Verification items for the finished model (mm, model axes). A direction names the side the tool comes from. Round coordinates to 2 decimals unless told otherwise and drop trailing zeros. Loops run counter-clockwise (first coordinate to the right, second up) from the corner with the lowest first, then second, coordinate; pieces in that order, holes last. Notation, with made-up numbers: M -12,12 L 38,12 A18 cw 38,28 Z; hole C -25,-19.75 d1. An arc over 180 degrees is marked long. Write item = value, one per line. Start each with the question number.
from build123d import *

# Parameters (mm, degrees)
BOSS_EXTRUDE1_DEPTH      = 46
SKETCH4_R                = 2.5
CUT_EXTRUDE2_DEPTH       = 49.124837662
CUT_EXTRUDE1_DEPTH       = 49.124837662
FILLET1_R                = 2
CIRPATTERN1_COUNT        = 4
FILLET1_OF_CIRPATTERN1_R = 2


with BuildPart() as part:
    # Sketch1 → Boss-Extrude1 (new body)
    with BuildSketch(Plane(origin=(0, 0, 0), x_dir=(1, 0, 0), z_dir=(0, 1, 0))):
        with BuildLine():
            Line((8.5, 10), (-8.5, 10))
            ThreePointArc((-8.5, 10), (-9.560660172, 9.560660172), (-10, 8.5))
            Line((-10, 8.5), (-10, -8.5))
            ThreePointArc((-10, -8.5), (-9.560660172, -9.560660172), (-8.5, -10))
            Line((-8.5, -10), (8.5, -10))
            ThreePointArc((8.5, -10), (9.560660172, -9.560660172), (10, -8.5))
            Line((10, -8.5), (10, 8.5))
            ThreePointArc((10, 8.5), (9.560660172, 9.560660172), (8.5, 10))
        make_face()
    extrude(amount=BOSS_EXTRUDE1_DEPTH)

    # Sketch4 → Cut-Extrude2 (cut, through all)
    with BuildSketch(Plane(origin=(0, 0, 0), x_dir=(1, 0, 0), z_dir=(0, 1, 0))):
        with Locations(Location((0, 0, 0), (0, 0, 270))):
            Circle(SKETCH4_R)
    extrude(amount=CUT_EXTRUDE2_DEPTH, mode=Mode.SUBTRACT)

    # Sketch2 → Cut-Extrude1 (cut, through all)
    with BuildSketch(Plane.XZ):
        Polygon((-3.6, -10), (-3.6, -9.5), (-3.1, -9.5), (-3.1, -8.2), (-5.5, -8.2), (-5.5, -6.560660172), (-2.839339828, -3.9), (2.839339828, -3.9), (5.5, -6.560660172), (5.5, -8.2), (3.1, -8.2), (3.1, -9.5), (3.6, -9.5), (3.6, -10), align=None)
    cut_extrude1 = extrude(amount=-CUT_EXTRUDE1_DEPTH, mode=Mode.SUBTRACT)

    # Fillet1
    fillet1_edges = [part.edges().sort_by_distance(p)[0] for p in [
        (-2.839339828, 23, -3.9),
        (2.839339828, 23, -3.9),
    ]]
    fillet(fillet1_edges, radius=FILLET1_R)

    # CirPattern1: Cut-Extrude1 ×4 about axis
    cirpattern1_axis = Axis((0, 0, 0), (0, 1, 0))
    for i in range(1, CIRPATTERN1_COUNT):
        add(cut_extrude1.rotate(cirpattern1_axis, i * 360 / CIRPATTERN1_COUNT), mode=Mode.SUBTRACT)

    # Fillet1 of CirPattern1
    fillet1_of_cirpattern1_edges = [part.edges().sort_by_distance(p)[0] for p in [
        (-3.9, 23, 2.839339828),
        (-3.9, 23, -2.839339828),
        (2.839339828, 23, 3.9),
        (-2.839339828, 23, 3.9),
        (3.9, 23, -2.839339828),
        (3.9, 23, 2.839339828),
    ]]
    fillet(fillet1_of_cirpattern1_edges, radius=FILLET1_OF_CIRPATTERN1_R)


solid = part.part
1. Tool access check on faces 4 (the cylindrical face through (4.05, 23.32, 2.77)), 5 (the flat face through (3.1, 23, 9)), 6 (the flat face through (-3.9, 23, 0)), 7 (the flat face through (9, 23, 3.1)). Record the directions out of +Z, -Z, +X, -X, +Y, -Y that give a thin tool (end or side, any length) a straight path to the whole face; none if there is none.
2. Thickness scan on line 1 (Z direction, x = 0, y = 28.5); line 2 (X direction, y = 24, z = -7.25). Record the ranges inside material, lowest first.
3. Section check B-B, the plane x = 0. Enter the section's corners in (y, z), and give its area (3 significant figures).
4. Section check A-A, the plane z = 0. Enter the section's corners in (x, y), and give its area (3 significant figures).
5. Mould release check, pull along Z, two halves, no side actions. Record for faces 1 (the flat face through (-10, 23, 6)), 2 (the cylindrical face through (2.77, 23.32, -4.05)), 3 (the flat face through (0, 23, -3.9)): pulls with the +Z half, pulls with the -Z half, needs draft (parallel to the pull), parting line crosses it, or undercut.
6. Gauge pin test, flat ends, axial feed: P1, Ø1.2, axis at x = 0, y = 12.5, coming from the -Z side; P2, Ø2, axis at y = 25, z = 0.5, coming from the +X side; P3, Ø0.6, axis at x = 3, y = 18.5, coming from the -Z side. Record the tip position at first contact, or that the pin passes through.
Computed values:
q1.face_4 = +Y, -Y
q1.face_5 = +Z, +Y, -Y
q1.face_6 = -X, +Y, -Y
q1.face_7 = +X, +Y, -Y
q2.line_1 = -3.9 to -2.5, 2.5 to 3.9
q2.line_2 = -10 to -5.5, 5.5 to 10
q3.outline = M 0,-3.9 L 46,-3.9 L 46,-2.5 L 0,-2.5 Z; M 0,2.5 L 46,2.5 L 46,3.9 L 0,3.9 Z
q3.area = 129 mm2
q4.outline = M -3.9,0 L -2.5,0 L -2.5,46 L -3.9,46 Z; M 2.5,0 L 3.9,0 L 3.9,46 L 2.5,46 Z
q4.area = 129 mm2
q5.face_1 = needs draft
q5.face_2 = undercut
q5.face_3 = pulls with the -Z half
q6.P1 = -3.9
q6.P2 = 3.9
q6.P3 = -9.5
